Part model, mm, in its own coordinate system. A direction names the side the tool comes from. Round coordinates to 2 decimals unless told otherwise and drop trailing zeros. Loops run counter-clockwise (first coordinate to the right, second up) from the corner with the lowest first, then second, coordinate; pieces in that order, holes last.
1) Band-saw the part on A-A, the plane x = 0. Write the cut outline in (y, z), then the cut area to 3 significant figures.
2) Band-saw the part on B-B, the plane z = 3. Write the cut outline in (x, y), then the cut area to 3 significant figures.
3) Band-saw the part on C-C, the plane z = 11.5. Write the cut outline in (x, y), then the cut area to 3 significant figures.
4) Probe line 1 (Y direction, x = 0, z = 12); line 2 (Y direction, x = 0, z = 5.5); line 3 (Y direction, x = 10, z = 14). List the from-to ranges inside material, lowest first.
5) 3-axis set-ups, long thin cutter, end or side, ignore diameter. For faces 1 (the cylindrical face through (6.691, -12.864, 12.726)), 2 (the conical face through (16, 0, 1)): which of +Z, -Z, +X, -X, +Y, -Y reach the whole face in a straight line?
6) Drop flat-ended pins along their axis: P1, Ø6, axis at y = 5.5, z = 1.5, coming from the +X side; P2, Ø9, axis at x = 1.5, y = -2, coming from the +Z side; P3, Ø10, axis at x = 1.5, y = 6.5, coming from the -Z side; P4, Ø1, axis at y = 6.5, z = 7, coming from the -X side. Give the stop position or say it passes through.
from build123d import *

# Parameters (mm, degrees)
ESQUISSE1_R                  = 17
CORPS_DE_MANOEUVRE_DEPTH     = 11
ESQUISSE2_R                  = 14.5
ORGANE_DE_FREIN_DEPTH        = 5
ESQUISSE3_R                  = 9.5
PER_AGE_DEPTH                = 29.879058156
CHANFREIN_DE_MANOEUVRE_SIZE  = 2
HEXAGON_INSCRIBED1_OUTSIDE_W = 46.136
HEXAGON_INSCRIBED1_OUTSIDE_H = 46.136
MANOEUVRE_DEPTH              = 39.920108467
CONG_1_R                     = 1.5
CHANFREIN2_SIZE              = 1


with BuildPart() as part:
    # Esquisse1 → corps de manoeuvre (new body)
    with BuildSketch(Plane.XY):
        Circle(ESQUISSE1_R)
    extrude(amount=CORPS_DE_MANOEUVRE_DEPTH)

    # Esquisse2 → organe de frein (add)
    with BuildSketch(Plane.XY.offset(11)):
        Circle(ESQUISSE2_R)
    extrude(amount=ORGANE_DE_FREIN_DEPTH)

    # Esquisse3 → perçage (cut, through all)
    with BuildSketch(Plane.XY.offset(16)):
        Circle(ESQUISSE3_R)
    extrude(amount=-PER_AGE_DEPTH, mode=Mode.SUBTRACT)

    # Chanfrein de manoeuvre
    chanfrein_de_manoeuvre_edges = [part.edges().sort_by_distance(p)[0] for p in [
        (-17, 0, 0),
        (-17, 0, 11),
    ]]
    chamfer(chanfrein_de_manoeuvre_edges, length=CHANFREIN_DE_MANOEUVRE_SIZE)

    # Hexagon - inscribed1 outside → manoeuvre (cut, through all)
    with BuildSketch(Plane(origin=(1.77823943, 13.102368129, 0), x_dir=(-1, 0, 0), z_dir=(0, 0, -1))):
        with Locations((1.778, -13.102)):
            Rectangle(HEXAGON_INSCRIBED1_OUTSIDE_W, HEXAGON_INSCRIBED1_OUTSIDE_H)
        Polygon((18.77823943, -13.102368129), (10.27823943, 1.620063735), (-6.72176057, 1.620063735), (-15.22176057, -13.102368129), (-6.72176057, -27.824799994), (10.27823943, -27.824799994), align=None, mode=Mode.SUBTRACT)
    extrude(amount=-MANOEUVRE_DEPTH, mode=Mode.SUBTRACT)

    # Congé1
    cong_1_edges = [part.edges().sort_by_distance(p)[0] for p in [
        (-14.5, 0, 16),
    ]]
    fillet(cong_1_edges, radius=CONG_1_R)

    # Chanfrein2
    chanfrein2_edges = [part.edges().sort_by_distance(p)[0] for p in [
        (-9.5, 0, 16),
        (-9.5, 0, 0),
    ]]
    chamfer(chanfrein2_edges, length=CHANFREIN2_SIZE)


solid = part.part
Reported:
1. outline: (-14.72, 0) - (-10.5, 0) - (-9.5, 1) - (-9.5, 15) - (-10.5, 16) - (-13, 16) arc R1.5 ccw to (-14.5, 14.5) - (-14.5, 11) - (-14.72, 11) - close; (9.5, 1) - (10.5, 0) - (14.72, 0) - (14.72, 11) - (14.5, 11) - (14.5, 14.5) arc R1.5 ccw to (13, 16) - (10.5, 16) - (9.5, 15) - close
1. area: 162 mm2
2. outline: (-17, 0) - (-8.5, -14.72) - (8.5, -14.72) - (17, 0) - (8.5, 14.72) - (-8.5, 14.72) - close; hole circle Ø19 at (0, 0)
2. area: 467 mm2
3. outline: circle Ø29 at (0, 0); hole circle Ø19 at (0, 0)
3. area: 377 mm2
4. line 1: y = -14.5 to -9.5, 9.5 to 14.5
4. line 2: y = -14.72 to -9.5, 9.5 to 14.72
4. line 3: y = -10.5 to 10.5
5. face 1: +Z
5. face 2: -Z, +X
6. P1: stops at x = 15.56
6. P2: passes through
6. P3: stops at z = 0
6. P4: stops at x = -13.54
